from build123d import *

# Parameters (mm, degrees)
F0_R     = 2.25
F0_R_2   = 4.5
F1_DEPTH = 4
F2_W     = 3.75
F2_H     = 5
F3_DEPTH = 3
F4_R     = 4.5
F5_DEPTH = 10


with BuildPart() as f1:
    # F0 (on Top) → F1 (new body)
    with BuildSketch(Plane.XY):
        with BuildLine():
            Line((-10, 35), (-10, 0))
            Line((-10, 0), (10, 0))
            Line((10, 0), (10, 35))
            ThreePointArc((10, 35), (0, 45), (-10, 35))
        make_face()
        with Locations((0, 11)):
            Circle(F0_R, mode=Mode.SUBTRACT)
        with Locations((0, 39.5)):
            Circle(F0_R_2, mode=Mode.SUBTRACT)
    extrude(amount=F1_DEPTH)

    # F2 (on Top) → F3 (join)
    with BuildSketch(Plane.XY):
        with Locations((-8.125, 11)):
            Rectangle(F2_W, F2_H)
        with Locations((8.125, 11)):
            Rectangle(F2_W, F2_H)
    extrude(amount=-F3_DEPTH)

    # F4 (on face) → F5 (join)
    with BuildSketch(Plane(origin=(0, 0, 0), x_dir=(1, 0, 0), z_dir=(0, 0, -1))):
        with BuildLine():
            ThreePointArc((2.4862908139, -44.6859877136), (4.8669921435, -42.5640656083), (5.7511834067, -39.5))
            ThreePointArc((5.7511834067, -39.5), (-3.0640656083, -34.6330078565), (-2.4862908139, -44.6859877136))
            ThreePointArc((-2.4862908139, -44.6859877136), (0, -45), (2.4862908139, -44.6859877136))
        make_face()
        with Locations((0, -39.5)):
            Circle(F4_R, mode=Mode.SUBTRACT)
        with BuildLine():
            ThreePointArc((2.4862908139, -44.6859877136), (0, -45), (-2.4862908139, -44.6859877136))
            ThreePointArc((-2.4862908139, -44.6859877136), (0, -45.2511834067), (2.4862908139, -44.6859877136))
        make_face()
    extrude(amount=-F5_DEPTH)


solid = f1.part
Could you check a few things on this model? Use its own coordinates, in mm. A direction names the side the tool comes from. Round coordinates to 2 decimals unless told otherwise and drop trailing zeros. Order: outer loops, then holes, each group sorted by start corner. A loop starts at its lowest first (then second) coordinate and runs counter-clockwise, first axis right, second up.
(1) I'm going to push flat-ended pins straight in: pin 1 (1 mm diameter, centred on x = -5.5, y = 26.5, fed in from +Z); pin 2 (4 mm diameter, centred on x = 0, y = 11, fed in from -Z); pin 3 (6 mm diameter, centred on x = 4.5, y = 28.5, fed in from -Z); pin 4 (2.5 mm diameter, centred on x = 8.5, z = -2, fed in from -Y). Where does each tip first touch, or does it pass through?
Response values:
pin 1: stops at z = 4
pin 2: passes through
pin 3: stops at z = 0
pin 4: stops at y = 8.5
(2) Imagine slicing it at D-D (z = 3.5). Write out the boundary of the cut face in (x, y).
Response values:
outline: (-10, 0) - (10, 0) - (10, 35) arc R10 ccw to (2.49, 44.69) arc R5.75 ccw to (-2.49, 44.69) arc R10 ccw to (-10, 35) - close; hole circle Ø9 at (0, 39.5); hole circle Ø4.5 at (0, 11)
(3) If we mould it in two halves opening along Y, with no side actions, what happens to faces 5 (the flat face through (8, 13.5, -1)), 6 (the cylindrical face through (-0.29, 13.23, 1.97)), 7 (the flat face through (10, 17, 1))? For each: released by +Y, released by -Y, zero draft, split by the parting line, or undercut.
Response values:
face 5: released by +Y
face 6: undercut
face 7: zero draft
(4) Imagine slicing it at A-A (x = 0). Write out the boundary of the cut face in (y, z).
Response values:
outline: (0, 0) - (8.75, 0) - (8.75, 4) - (0, 4) - close; (13.25, 0) - (35, 0) - (35, 10) - (33.75, 10) - (33.75, 4) - (13.25, 4) - close; (44, 0) - (45.25, 0) - (45.25, 10) - (44, 10) - close
(5) Imagine slicing it at B-B (z = -0.5). Write out the boundary of the cut face in (x, y), plus the area to 3 significant figures.
Response values:
outline: (-10, 8.5) - (-6.25, 8.5) - (-6.25, 13.5) - (-10, 13.5) - close; (6.25, 8.5) - (10, 8.5) - (10, 13.5) - (6.25, 13.5) - close
area: 37.5 mm2
(6) Imagine slicing it at C-C (y = 11). Write out the boundary of the cut face in (x, z).
Response values:
outline: (-10, -3) - (-6.25, -3) - (-6.25, 0) - (-2.25, 0) - (-2.25, 4) - (-10, 4) - close; (2.25, 0) - (6.25, 0) - (6.25, -3) - (10, -3) - (10, 4) - (2.25, 4) - close
(7) Which directions (+Z, -Z, +X, -X, +Y, -Y) give clear straight access to the entire face, cutting with the end or side of a thin tool? Please do faces 1 (the flat face through (-8, 13.5, -1)), 2 (the flat face through (6.25, 11, -1)), 3 (the cylindrical face through (8, 41, 2)), 4 (the flat face through (8, 8.5, -1)).
Response values:
face 1: -Z, +X, -X, +Y
face 2: -Z, +Y, -Y
face 3: +Z, -Z, +X, +Y
face 4: -Z, +X, -X, -Y
(8) Please list where these lines run through material, in increasing order: line 1 along Y through (x, z) = (0.5, 1); line 2 along X through (y, z) = (9, -0.5); line 3 along Y through (x, z) = (0.75, 3).
Response values:
line 1: y = 0 to 8.81, 13.19 to 35.03, 43.97 to 45.23
line 2: x = -10 to -6.25, 6.25 to 10
line 3: y = 0 to 8.88, 13.12 to 35.06, 43.94 to 45.2
